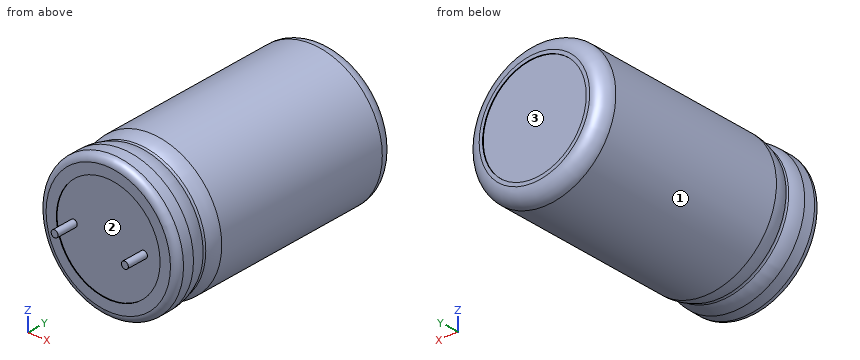
from build123d import *

# Parameters (mm, degrees)
SKETCH1_R           = 0.5
BASE_EXTRUDE_DEPTH  = 3
SKETCH2_R           = 7.5
BOSS_EXTRUDE1_DEPTH = 0.690752369
SKETCH3_R           = 0.5
BOSS_EXTRUDE2_DEPTH = 3
SKETCH4_R           = 10
BOSS_EXTRUDE3_DEPTH = 35.2
SKETCH5_R           = 7.5
SKETCH5_R_2         = 0.5
CUT_EXTRUDE1_DEPTH  = 0.1
FILLET1_R           = 2
FILLET2_R           = 1
SKETCH7_R           = 7.5
CUT_EXTRUDE2_DEPTH  = 0.1


with BuildPart() as part:
    # Sketch1 → Base-Extrude (new body)
    with BuildSketch(Plane(origin=(0, 0, 0), x_dir=(1, 0, 0), z_dir=(0, 1, 0))):
        Circle(SKETCH1_R)
    extrude(amount=-BASE_EXTRUDE_DEPTH)

    # Sketch2 → Boss-Extrude1 (add)
    with BuildSketch(Plane(origin=(0, 0, 0), x_dir=(1, 0, 0), z_dir=(0, 1, 0))):
        with Locations((-5.08, 0)):
            Circle(SKETCH2_R)
    extrude(amount=BOSS_EXTRUDE1_DEPTH)

    # Sketch3 → Boss-Extrude2 (add)
    with BuildSketch(Plane.XZ):
        with Locations((-10.16, 0)):
            Circle(SKETCH3_R)
    extrude(amount=BOSS_EXTRUDE2_DEPTH)

    # Sketch4 → Boss-Extrude3 (add)
    with BuildSketch(Plane.XZ):
        with Locations((-5.08, 0)):
            Circle(SKETCH4_R)
    extrude(amount=-BOSS_EXTRUDE3_DEPTH)

    # Sketch5 → Cut-Extrude1 (cut)
    with BuildSketch(Plane.XZ):
        with Locations((-5.08, 0)):
            Circle(SKETCH5_R)
        Circle(SKETCH5_R_2, mode=Mode.SUBTRACT)
        with Locations((-10.16, 0)):
            Circle(SKETCH5_R_2, mode=Mode.SUBTRACT)
    extrude(amount=-CUT_EXTRUDE1_DEPTH, mode=Mode.SUBTRACT)

    # Fillet1
    fillet1_edges = [part.edges().sort_by_distance(p)[0] for p in [
        (-15.08, 35.2, 0),
    ]]
    fillet(fillet1_edges, radius=FILLET1_R)

    # Fillet2
    fillet2_edges = [part.edges().sort_by_distance(p)[0] for p in [
        (-15.08, 0, 0),
    ]]
    fillet(fillet2_edges, radius=FILLET2_R)

    # Sketch6 → Cut-Revolve1 (revolve, cut)
    with BuildSketch(Plane.XY):
        with BuildLine():
            Line((4.92, 7.19), (5.42, 7.19))
            Line((5.42, 7.19), (5.42, 2.61))
            Line((5.42, 2.61), (4.92, 2.61))
            ThreePointArc((4.92, 2.61), (4.804920837, 3.674592058), (4.465, 4.69))
            ThreePointArc((4.465, 4.69), (4.398803332, 4.9), (4.465, 5.11))
            ThreePointArc((4.465, 5.11), (4.804920837, 6.125407942), (4.92, 7.19))
        make_face()
    revolve(axis=Axis((-5.08, 0, 0), (0, 1, 0)), mode=Mode.SUBTRACT)

    # Sketch7 → Cut-Extrude2 (cut)
    with BuildSketch(Plane(origin=(0, 35.2, 0), x_dir=(-1, 0, 0), z_dir=(0, 1, 0))):
        with Locations((5.08, 0)):
            Circle(SKETCH7_R)
    extrude(amount=-CUT_EXTRUDE2_DEPTH, mode=Mode.SUBTRACT)


solid = part.part
Here's how the part is built. I have some questions about the finished solid (model axes, mm). Face numbers are marked on the shaded views. Round coordinates to 2 decimals unless told otherwise and drop trailing zeros. Order: outer loops, then holes, each group sorted by start corner. A loop starts at its lowest first (then second) coordinate and runs counter-clockwise, first axis right, second up. Notation, with made-up numbers: M -34.5,72 L 7.5,72 A32 ccw 7.5,108 Z; hole C 49.25,42.5 d10. An arc over 180 degrees is marked long. Return JSON: item names as keys, results as strings. Group by question number.
1. Please list where these lines run through material, in increasing order: probe 1 along Y at (x, z) = (-10.25, -3); probe 2 along Y at (x, z) = (-3.5, 8); probe 3 along Z at (x, y) = (-1, 15).
2. I'm going to push flat-ended pins straight in: pin 1 Ø4 at (x, y) = (-7.5, 10) entering from -Z; pin 2 Ø1.5 at (y, z) = (9.5, -7) entering from +X; pin 3 Ø5 at (x, y) = (2.5, 14) entering from +Z. Where does each tip first touch, or does it pass through?
3. If we section it at C-C on y = 22: List the corners of the cut face in (x, z) for me.
4. If we section it at A-A on x = -5.08: List the corners of the cut face in (y, z) for me (3 decimals).
5. If we mould it in two halves opening along Z, with no side actions, what happens to the marked faces 1, 2 and 3? For each: pulls with the +Z half, pulls with the -Z half, needs draft (parallel to the pull), parting line crosses it, or undercut.
Reply:
{
 "1": {"probe 1": "0.1 to 35.1", "probe 2": "0 to 35.19", "probe 3": "-9.13 to 9.13"},
 "2": {"pin 1": "z = -9.99", "pin 2": "x = 2.73", "pin 3": "z = 8.61"},
 "3": {"outline": "C -5.08,0 d20"},
 "4": {"outline": "M 0,-9 A1 ccw 1,-10 L 2.61,-10 A4.982 ccw 4.69,-9.545 A0.366 cw 5.11,-9.545 A4.982 ccw 7.19,-10 L 33.2,-10 A2 ccw 35.2,-8 L 35.2,-7.5 L 35.1,-7.5 L 35.1,7.5 L 35.2,7.5 L 35.2,8 A2 ccw 33.2,10 L 7.19,10 A4.982 ccw 5.11,9.545 A0.366 cw 4.69,9.545 A4.982 ccw 2.61,10 L 1,10 A1 ccw 0,9 L 0,7.5 L 0.1,7.5 L 0.1,-7.5 L 0,-7.5 Z"},
 "5": {"face 1": "parting line crosses it", "face 2": "undercut", "face 3": "undercut"}
}
